```python
from build123d import *

# Parameters (mm, degrees)
SKETCH1_W                = 182
SKETCH1_H                = 150.75023901
SKETCH1_R                = 1.5
BOSS_EXTRUDE1_DEPTH      = 3
SKETCH2_R                = 4
SKETCH2_R_2              = 1.5
BOSS_EXTRUDE2_DEPTH      = 10
BOSS_EXTRUDE2_DEPTH_BACK = 25


with BuildPart() as part:
    # Sketch1 → Boss-Extrude1 (new body)
    with BuildSketch(Plane(origin=(0, 0, 0), x_dir=(1, 0, 0), z_dir=(0, 1, 0))):
        with Locations((81, 65.375119505)):
            Rectangle(SKETCH1_W, SKETCH1_H)
        with Locations((0, 130.75023901)):
            Circle(SKETCH1_R, mode=Mode.SUBTRACT)
        with Locations((162, 130.75023901)):
            Circle(SKETCH1_R, mode=Mode.SUBTRACT)
        with Locations((162, 0)):
            Circle(SKETCH1_R, mode=Mode.SUBTRACT)
        Circle(SKETCH1_R, mode=Mode.SUBTRACT)
    extrude(amount=BOSS_EXTRUDE1_DEPTH)

    # Sketch2 → Boss-Extrude2 (add, two sides)
    with BuildSketch(Plane(origin=(0, 3, 0), x_dir=(1, 0, 0), z_dir=(0, 1, 0))) as boss_extrude2_sk:
        with Locations((0, 130.75023901)):
            Circle(SKETCH2_R)
        with Locations((0, 130.75023901)):
            Circle(SKETCH2_R_2, mode=Mode.SUBTRACT)
        with Locations((162, 130.75023901)):
            Circle(SKETCH2_R)
        with Locations((162, 130.75023901)):
            Circle(SKETCH2_R_2, mode=Mode.SUBTRACT)
        with Locations((162, 0)):
            Circle(SKETCH2_R)
        with Locations((162, 0)):
            Circle(SKETCH2_R_2, mode=Mode.SUBTRACT)
        Circle(SKETCH2_R)
        Circle(SKETCH2_R_2, mode=Mode.SUBTRACT)
    extrude(amount=BOSS_EXTRUDE2_DEPTH)
    extrude(boss_extrude2_sk.sketch, amount=-BOSS_EXTRUDE2_DEPTH_BACK)


solid = part.part
```
Source: CAD feature listing. Evaluate the final solid. Frame: model axes, mm. A direction names the side the tool comes from. Give positions to 0.01 mm unless a question says otherwise; leave off trailing zeros. Write each loop counter-clockwise with the first axis right and the second up, starting at its lowest first coordinate (ties: lowest second). Pieces come first, ordered by that corner, then holes. Notation, with made-up numbers: (45, 24) - (56, 24) arc R29 cw to (56, 53) - close; hole circle Ø6 at (6.5, 10.25). An arc over 180 degrees is marked (long way). One line per item, written item: value. Start each with the question number.
Q1. Draft query along X for faces 1 (the face through (164, 13, -131)), 2 (the face through (-0.867, -10.846, 3.905)). Return one class per face: +X half, -X half, draft (parallel to the pull), parting line (faces both ways), or undercut.
Q2. Material intervals for probe 1 along X at (y, z) = (-6, 0); probe 2 along X at (y, z) = (0.85, 0); probe 3 along Z at (x, y) = (0, 6), sorted ascending. Write a range as from..to.
Q3. Section query B-B, the plane x = 62.5. Return the cut outline in (y, z).
Q4. Set-up query: faces 3 (the face through (-0.867, 7.93, 3.905)), 4 (the face through (80, 0, -66)), 5 (the face through (2, 13, 0)). Return all of +Z, -Z, +X, -X, +Y, -Y with unobstructed straight access to the full face (end or side cutting, diameter ignored); none if empty.
Q5. Section query A-A, the plane y = 10. Return the cut outline in (x, z).
Q6. Section query C-C, the plane z = -56.5. Return the cut outline in (x, y).
Q7. First-contact query: pin 1 Ø5 at (x, z) = (30, -70.5) entering from +Y; pin 2 Ø6 at (x, z) = (124.5, -76) entering from -Y. Flat tips, straight axial feed; report the tip coordinate or a pass-through.
Answer:
1. face 1: draft
1. face 2: undercut
2. probe 1: x = -4..-1.5, 1.5..4, 158..160.5, 163.5..166
2. probe 2: x = -10..-1.5, 1.5..160.5, 163.5..172
2. probe 3: z = -134.75..-132.25, -129.25..-126.75, -4..-1.5, 1.5..4
3. outline: (0, -140.75) - (3, -140.75) - (3, 10) - (0, 10) - close
4. face 3: +Y
4. face 4: -Y
4. face 5: +Z, -Z, +X, -X, +Y
5. outline: circle Ø8 at (0, -130.75); circle Ø8 at (0, 0); circle Ø8 at (162, -130.75); circle Ø8 at (162, 0); hole circle Ø3 at (0, -130.75); hole circle Ø3 at (0, 0); hole circle Ø3 at (162, -130.75); hole circle Ø3 at (162, 0)
6. outline: (-10, 0) - (172, 0) - (172, 3) - (-10, 3) - close
7. pin 1: stops at y = 3
7. pin 2: stops at y = 0
